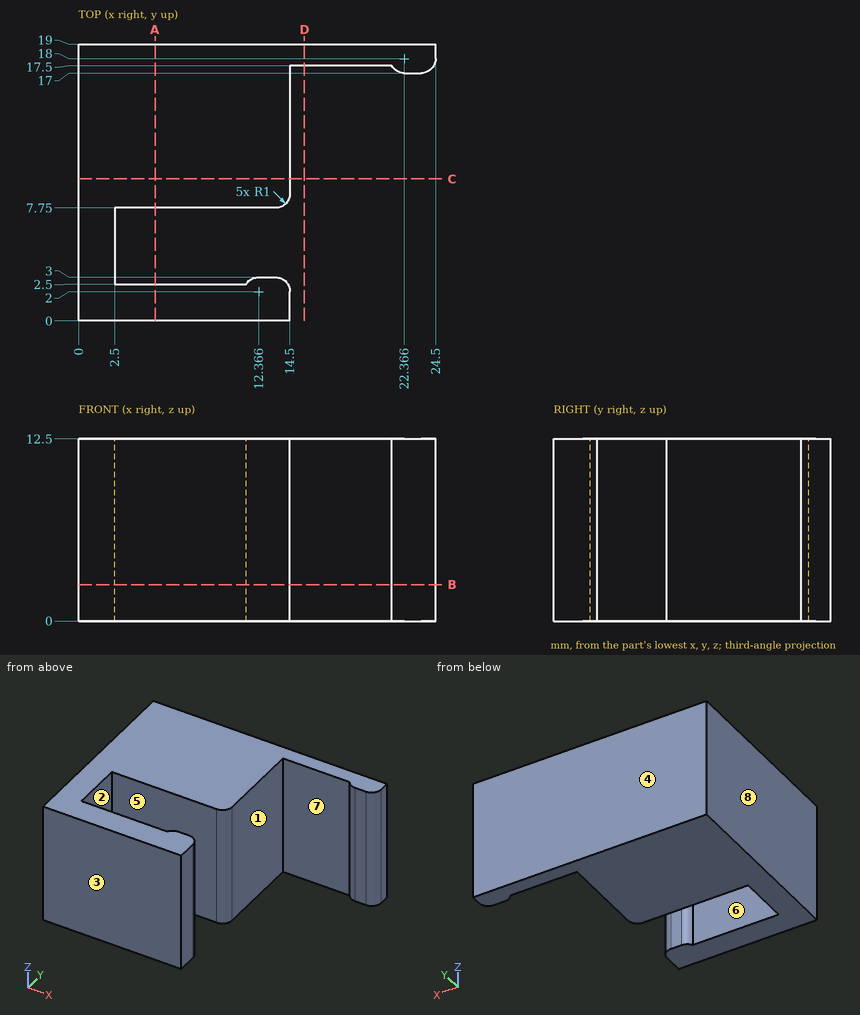
The drawing under review shows one solid part. Ordinate dimensions are in mm from its lowest x, y, z. A direction names the side the tool comes from. Give positions to 0.01 mm unless a question says otherwise; leave off trailing zeros. Write each loop counter-clockwise with the first axis right and the second up, starting at its lowest first coordinate (ties: lowest second). Pieces come first, ordered by that corner, then holes.
1. Draft analysis for pull direction Y (two halves, no side actions). For the marked faces 1, 2 and 3, state which applies: +Y half, -Y half, draft (parallel to the pull), parting line (faces both ways), or undercut.
2. Add section A-A, the plane x = 5.25. Write out the cut boundary in (y, z).
3. Tool access review of the marked faces 4, 5, 6, 7 and 8: name each direction out of +Z, -Z, +X, -X, +Y, -Y from which nothing blocks a thin tool from reaching the whole face with its end or side.
4. Add section D-D, the plane x = 15.5. Write out the cut boundary in (y, z), plus the area to 4 significant figures.
5. For P1, Ø2.5, axis at y = 4, z = 5.5, coming from the +X side; P2, Ø0.6, axis at x = 23, z = 9, coming from the -Y side; P3, Ø2, axis at y = 3, z = 11, coming from the +X side, all flat-tipped, find the tip position at first contact; note any pin that passes through.
6. Add section C-C, the plane y = 9.75. Write out the cut boundary in (x, z).
7. Wall thickness on L1, parallel to Y at x = 7, z = 2; L2, parallel to X at y = 12.25, z = 3.25; L3, parallel to Y at x = 22.5, z = 11.5: over which ranges is each line inside the solid? List them lowest first.
8. Add section B-B, the plane z = 2.5. Write out the cut boundary in (x, y).
Worked answers:
1. face 1: draft
1. face 2: undercut
1. face 3: -Y half
2. outline: (0, 0) - (2.5, 0) - (2.5, 12.5) - (0, 12.5) - close; (7.75, 0) - (19, 0) - (19, 12.5) - (7.75, 12.5) - close
3. face 4: +Z, -Z, +X, -X, +Y
3. face 5: +Z, -Z, +X
3. face 6: +Z, -Z
3. face 7: +Z, -Z, -Y
3. face 8: +Z, -Z, -X, +Y, -Y
4. outline: (17.5, 0) - (19, 0) - (19, 12.5) - (17.5, 12.5) - close
4. area: 18.75 mm2
5. P1: stops at x = 14.16
5. P2: stops at y = 17
5. P3: stops at x = 14.5
6. outline: (0, 0) - (14.5, 0) - (14.5, 12.5) - (0, 12.5) - close
7. L1: y = 0 to 2.5, 7.75 to 19
7. L2: x = 0 to 14.5
7. L3: y = 17 to 19
8. outline: (0, 0) - (14.5, 0) - (14.5, 2) arc R1 ccw to (13.5, 3) - (12.37, 3) arc R1 ccw to (11.5, 2.5) - (2.5, 2.5) - (2.5, 7.75) - (13.5, 7.75) arc R1 ccw to (14.5, 8.75) - (14.5, 17.5) - (21.5, 17.5) arc R1 ccw to (22.37, 17) - (23.5, 17) arc R1 ccw to (24.5, 18) - (24.5, 19) - (0, 19) - close
